Design review of the part built by this model. Coordinates are the model's own, in mm. Coordinates: 2 decimals unless noted, no trailing zeros. Write each loop counter-clockwise with the first axis right and the second up, starting at its lowest first coordinate (ties: lowest second). Pieces come first, ordered by that corner, then holes.
Q1. Add section C-C, the plane y = 0.75. Give the boundary of the cut face in (x, z).
Q2. The part is to be moulded in two halves that separate along X. For faces 1 (the face through (0, 3, -2.05)), 2 (the face through (-2.8, 3.5, 0)), 3 (the face through (2.8, 3.5, 0)), 4 (the face through (-1.16, 3.45, -0.37)), say which applies: +X half, -X half, draft (parallel to the pull), parting line (faces both ways), or undercut.
Q3. Add section A-A, the plane x = 0. Give the boundary of the cut face in (y, z), plus the area to 3 significant figures.
Q4. Add section B-B, the plane z = 0. Give the boundary of the cut face in (x, y).
Q5. To check wall thickness, follow probe 1 along Z at (x, y) = (0, 2.5); probe 2 along X at (y, z) = (2.75, -0.9); probe 3 along X at (y, z) = (1.5, 1). State the ranges of each line that lie inside material, in increasing order.
from build123d import *

# Parameters (mm, degrees)
BOSS_EXTRUDE1_DEPTH   = 7
F_2_CLEARANCE_HOLE1_D = 2.4384


with BuildPart() as part:
    # Sketch1 → Boss-Extrude1 (new body)
    with BuildSketch(Plane(origin=(0, 0, 0), x_dir=(1, 0, 0), z_dir=(0, 1, 0))):
        with BuildLine():
            Line((-1.907223112, 2.05), (1.907223112, 2.05))
            ThreePointArc((1.907223112, 2.05), (2.8, 0), (1.907223112, -2.05))
            Line((1.907223112, -2.05), (-1.907223112, -2.05))
            ThreePointArc((-1.907223112, -2.05), (-2.8, 0), (-1.907223112, 2.05))
        make_face()
    extrude(amount=BOSS_EXTRUDE1_DEPTH)

    # #2 Clearance Hole1 (through all)
    with Locations(Plane(origin=(0, 7, 0), x_dir=(1, 0, 0), z_dir=(0, 1, 0))):
        with Locations((0, 0)):
            Hole(F_2_CLEARANCE_HOLE1_D / 2)


solid = part.part
Here are the results:
1. outline: (-1.91, -2.05) - (1.91, -2.05) arc R2.8 ccw to (1.91, 2.05) - (-1.91, 2.05) arc R2.8 ccw to start; hole circle Ø2.44 at (0, 0)
2. face 1: draft
2. face 2: -X half
2. face 3: +X half
2. face 4: undercut
3. outline: (0, -2.05) - (7, -2.05) - (7, -1.22) - (0, -1.22) - close; (0, 1.22) - (7, 1.22) - (7, 2.05) - (0, 2.05) - close
3. area: 11.6 mm2
4. outline: (-2.8, 0) - (-1.22, 0) - (-1.22, 7) - (-2.8, 7) - close; (1.22, 0) - (2.8, 0) - (2.8, 7) - (1.22, 7) - close
5. probe 1: z = -2.05 to -1.22, 1.22 to 2.05
5. probe 2: x = -2.65 to -0.82, 0.82 to 2.65
5. probe 3: x = -2.62 to -0.7, 0.7 to 2.62
